Can you work these out from the model? Positions are in its coordinate system, mm. A direction names the side the tool comes from. Round coordinates to 2 decimals unless told otherwise and drop trailing zeros. Loops run counter-clockwise (first coordinate to the right, second up) from the corner with the lowest first, then second, coordinate; pieces in that order, holes last. Notation, with made-up numbers: (6, 26) -> (13, 26) arc R33 cw to (13, 58) -> close; hole circle Ø5 at (24.5, 60.25). An arc over 180 degrees is marked (long way). Use a Markdown table: item, result.
from build123d import *

# Parameters (mm, degrees)
CUT_EXTRUDE1_REACH = 12
SKETCH2_R          = 4
CUT_EXTRUDE2_DEPTH = 4
CHAMFER1_SIZE      = 0.75


with BuildPart() as part:
    # Sketch1 → Revolve1 (revolve)
    with BuildSketch(Plane.XY):
        Polygon((0, 0), (-49, 0), (-49, 10), (-12, 10), (-12, 36), (0, 36), align=None)
    revolve(axis=Axis((0, 36, 0), (0, -1, 0)))

    # Sketch2 → Cut-Extrude1 (cut, up to next)
    with BuildSketch(Plane(origin=(0, 10, 0), x_dir=(1, 0, 0), z_dir=(0, 1, 0)), mode=Mode.PRIVATE) as cut_extrude1_sk1:
        with Locations((-28.284271247, 28.284271247)):
            Circle(SKETCH2_R)
    cut_extrude1_tool1 = extrude(cut_extrude1_sk1.sketch, amount=-CUT_EXTRUDE1_REACH, mode=Mode.PRIVATE) & part.part
    add(cut_extrude1_tool1.solids().sort_by_distance((-28.284271, 10, -28.284271))[0], mode=Mode.SUBTRACT)
    # Sketch2 → Cut-Extrude1 (cut, up to next)
    with BuildSketch(Plane(origin=(0, 10, 0), x_dir=(1, 0, 0), z_dir=(0, 1, 0)), mode=Mode.PRIVATE) as cut_extrude1_sk2:
        with Locations((28.284271247, 28.284271247)):
            Circle(SKETCH2_R)
    cut_extrude1_tool2 = extrude(cut_extrude1_sk2.sketch, amount=-CUT_EXTRUDE1_REACH, mode=Mode.PRIVATE) & part.part
    add(cut_extrude1_tool2.solids().sort_by_distance((28.284271, 10, -28.284271))[0], mode=Mode.SUBTRACT)
    # Sketch2 → Cut-Extrude1 (cut, up to next)
    with BuildSketch(Plane(origin=(0, 10, 0), x_dir=(1, 0, 0), z_dir=(0, 1, 0)), mode=Mode.PRIVATE) as cut_extrude1_sk3:
        with Locations((28.284271247, -28.284271247)):
            Circle(SKETCH2_R)
    cut_extrude1_tool3 = extrude(cut_extrude1_sk3.sketch, amount=-CUT_EXTRUDE1_REACH, mode=Mode.PRIVATE) & part.part
    add(cut_extrude1_tool3.solids().sort_by_distance((28.284271, 10, 28.284271))[0], mode=Mode.SUBTRACT)
    # Sketch2 → Cut-Extrude1 (cut, up to next)
    with BuildSketch(Plane(origin=(0, 10, 0), x_dir=(1, 0, 0), z_dir=(0, 1, 0)), mode=Mode.PRIVATE) as cut_extrude1_sk4:
        with Locations((-28.284271247, -28.284271247)):
            Circle(SKETCH2_R)
    cut_extrude1_tool4 = extrude(cut_extrude1_sk4.sketch, amount=-CUT_EXTRUDE1_REACH, mode=Mode.PRIVATE) & part.part
    add(cut_extrude1_tool4.solids().sort_by_distance((-28.284271, 10, 28.284271))[0], mode=Mode.SUBTRACT)

    # Sketch3 → Cut-Extrude2 (cut)
    with BuildSketch(Plane.XY.offset(12)):
        with BuildLine():
            Line((-4, 36), (4, 36))
            Line((4, 36), (4, 16))
            ThreePointArc((4, 16), (0, 12), (-4, 16))
            Line((-4, 16), (-4, 36))
        make_face()
    extrude(amount=-CUT_EXTRUDE2_DEPTH, mode=Mode.SUBTRACT)

    # Chamfer1
    chamfer1_edges = [part.edges().sort_by_distance(p)[0] for p in [
        (6.92820323, 36, -9.797958971),
        (49, 10, 0),
        (49, 0, 0),
    ]]
    chamfer(chamfer1_edges, length=CHAMFER1_SIZE)


solid = part.part
1. If we mould it in two halves opening along Z, with no side actions, what happens to faces 3 (the cylindrical face through (31.979, 5.07, 29.816)), 4 (the flat face through (-10, 10, 10)), 5 (the cylindrical face through (1.56, 22.8, -11.9))? For each: +Z half, -Z half, draft (parallel to the pull), parting line (faces both ways), or undercut.
Answer sheet:
| item | result |
|---|---|
| face 3 | undercut |
| face 4 | draft |
| face 5 | parting line |
2. Which directions (+Z, -Z, +X, -X, +Y, -Y) give clear straight access to the entire face, cutting with the end or side of a thin tool? Please do faces 1 (the flat face through (0, 36, -1)), 2 (the flat face through (4, 26, 10)).
Answer sheet:
| item | result |
|---|---|
| face 1 | +Z, -Z, +X, -X, +Y |
| face 2 | +Z, +Y |
3. I want a section at A-A (x = 0). Please give me the cut outline in (y, z).
Answer sheet:
| item | result |
|---|---|
| outline | (0, -48.25) -> (0.75, -49) -> (9.25, -49) -> (10, -48.25) -> (10, -12) -> (35.25, -12) -> (36, -11.25) -> (36, 8) -> (12, 8) -> (12, 12) -> (10, 12) -> (10, 48.25) -> (9.25, 49) -> (0.75, 49) -> (0, 48.25) -> close |
4. Will these pins go through, and if not, where does the flat tip stop? pin 1 Ø9 at (x, y) = (-0.5, 18.5) entering from +Z; pin 2 Ø4 at (x, y) = (20.5, 11) entering from +Z; pin 3 Ø6 at (y, z) = (23, 3.5) entering from +X.
Answer sheet:
| item | result |
|---|---|
| pin 1 | stops at z = 11.32 |
| pin 2 | stops at z = 44.94 |
| pin 3 | stops at x = 11.99 |
5. I want a section at D-D (y = 25.5). Please give me the cut outline in (x, z), plus the area to 3 significant figures.
Answer sheet:
| item | result |
|---|---|
| outline | (-4, 8) -> (-4, 11.31) arc R12 ccw (long way) to (4, 11.31) -> (4, 8) -> close |
| area | 422 mm² |
6. I want a section at B-B (z = 0). Please give me the cut outline in (x, y), plus the area to 3 significant figures.
Answer sheet:
| item | result |
|---|---|
| outline | (-49, 0.75) -> (-48.25, 0) -> (48.25, 0) -> (49, 0.75) -> (49, 9.25) -> (48.25, 10) -> (12, 10) -> (12, 35.25) -> (11.25, 36) -> (-11.25, 36) -> (-12, 35.25) -> (-12, 10) -> (-48.25, 10) -> (-49, 9.25) -> close |
| area | 1,600 mm² |
7. I want a section at C-C (y = 5). Please give me the cut outline in (x, z), plus the area to 3 significant figures.
Answer sheet:
| item | result |
|---|---|
| outline | circle Ø98 at (0, 0); hole circle Ø8 at (-28.28, -28.28); hole circle Ø8 at (-28.28, 28.28); hole circle Ø8 at (28.28, -28.28); hole circle Ø8 at (28.28, 28.28) |
| area | 7,340 mm² |
8. I need wall thicknesses on line 1 (Y direction, x = -8, z = 37); line 2 (X direction, y = 7, z = -31.5); line 3 (X direction, y = 32, z = 0). Which ranges of each line are inside material? Lowest first, please.
Answer sheet:
| item | result |
|---|---|
| line 1 | y = 0 to 10 |
| line 2 | x = -37.53 to -30.66, -25.91 to 25.91, 30.66 to 37.53 |
| line 3 | x = -12 to 12 |
